from build123d import *

# Parameters (mm, degrees)
SKETCH1_R               = 20
SKETCH1_R_2             = 16
BOSS_EXTRUDE1_DEPTH     = 100
CUT_EXTRUDE1_DEPTH      = 52
CUT_EXTRUDE1_DEPTH_BACK = 46
SKETCH2_R               = 1.575


with BuildPart() as part:
    # Sketch1 → Boss-Extrude1 (new body)
    with BuildSketch(Plane(origin=(0, 0, 0), x_dir=(1, 0, 0), z_dir=(0, 1, 0))):
        with Locations(Location((0, 0, 0), (0, 0, 270))):
            Circle(SKETCH1_R)
        with Locations(Location((0, 0, 0), (0, 0, 270))):
            Circle(SKETCH1_R_2, mode=Mode.SUBTRACT)
    extrude(amount=BOSS_EXTRUDE1_DEPTH)

    # Sketch2 → Cut-Extrude1 (cut, two sides: drawn at the far end of the back side and taken through both)
    with BuildSketch(Plane(origin=(0, 0, 0), x_dir=(0, 0, -1), z_dir=(1, 0, 0)).offset(-CUT_EXTRUDE1_DEPTH_BACK)):
        with Locations(Location((0, 95, 0), (0, 0, 180))):
            Circle(SKETCH2_R)
        with Locations(Location((0, 5, 0), (0, 0, 180))):
            Circle(SKETCH2_R)
    extrude(amount=CUT_EXTRUDE1_DEPTH + CUT_EXTRUDE1_DEPTH_BACK, mode=Mode.SUBTRACT)


solid = part.part
Geometry: final body of the model. Coordinates: model frame, mm. Coordinates: 2 decimals unless noted, no trailing zeros. Order: outer loops, then holes, each group sorted by start corner. A loop starts at its lowest first (then second) coordinate and runs counter-clockwise, first axis right, second up.
1) Section A-A (x = 0). Return loops of the section in (y, z).
Result sheet:
outline: (0, -20) - (100, -20) - (100, -16) - (0, -16) - close; (0, 16) - (100, 16) - (100, 20) - (0, 20) - close
2) Section C-C (y = 5). Return loops of the section in (x, z) (3 decimals), then the cut area to 3 significant figures.
Result sheet:
outline: (-19.938, -1.575) arc R20 ccw to (19.938, -1.575) - (15.922, -1.575) arc R16 cw to (-15.922, -1.575) - close; (-19.938, 1.575) - (-15.922, 1.575) arc R16 cw to (15.922, 1.575) - (19.938, 1.575) arc R20 ccw to start
area: 427 mm2
3) Section D-D (y = 16). Return loops of the section in (x, z).
Result sheet:
outline: circle Ø40 at (0, 0); hole circle Ø32 at (0, 0)
4) First-contact query: P1, Ø1, axis at y = 67, z = 3, coming from the +X side; P2, Ø2, axis at y = 22, z = 5.5, coming from the +X side; P3, Ø3, axis at y = 70.5, z = -3.5, coming from the +X side. Flat tips, straight axial feed; report the tip coordinate or a pass-through.
Result sheet:
P1: stops at x = 19.84
P2: stops at x = 19.49
P3: stops at x = 19.9
5) Ray query, probe 1 along Y at (x, z) = (-18.5, 0) (3 decimals); probe 2 along X at (y, z) = (38.5, 0); probe 3 along X at (y, z) = (33.5, -13). Return the intervals inside material, ascending.
Result sheet:
probe 1: y = 0 to 3.425, 6.575 to 93.425, 96.575 to 100
probe 2: x = -20 to -16, 16 to 20
probe 3: x = -15.2 to -9.33, 9.33 to 15.2
6) Draft query along X for faces 1 (the cylindrical face through (-15.62, 49.3, -3.47)), 2 (the cylindrical face through (-19.524, 49.3, -4.336)), 3 (the cylindrical face through (17.93, 3.44, -0.21)). Return one class per face: released by +X, released by -X, zero draft, split by the parting line, or undercut.
Result sheet:
face 1: undercut
face 2: split by the parting line
face 3: zero draft
7) Section B-B (z = 0). Return loops of the section in (x, y) (3 decimals), then the cut area to 3 significant figures.
Result sheet:
outline: (-20, 0) - (-16, 0) - (-16, 3.425) - (-20, 3.425) - close; (-20, 6.575) - (-16, 6.575) - (-16, 93.425) - (-20, 93.425) - close; (-20, 96.575) - (-16, 96.575) - (-16, 100) - (-20, 100) - close; (16, 0) - (20, 0) - (20, 3.425) - (16, 3.425) - close; (16, 6.575) - (20, 6.575) - (20, 93.425) - (16, 93.425) - close; (16, 96.575) - (20, 96.575) - (20, 100) - (16, 100) - close
area: 750 mm2
